```python
from build123d import *

# Parameters (mm, degrees)
SCHIZZO1_W                   = 35.5
SCHIZZO1_H                   = 64
ESTRUSIONE_ESTRUSIONE1_DEPTH = 1
SCHIZZO2_W                   = 13
SCHIZZO2_H                   = 23
ESTRUSIONE_ESTRUSIONE2_DEPTH = 2.5
SCHIZZO3_R                   = 0.51
TAGLIO_ESTRUSIONE1_DEPTH     = 2.5
ESTRUSIONE_ESTRUSIONE3_DEPTH = 7
TAGLIO_ESTRUSIONE2_DEPTH     = 6
SCHIZZO7_R                   = 1.15
TAGLIO_ESTRUSIONE3_DEPTH     = 6


with BuildPart() as part:
    # Schizzo1 → Estrusione-Estrusione1 (new body)
    with BuildSketch(Plane(origin=(0, 0, 0), x_dir=(1, 0, 0), z_dir=(0, 1, 0))):
        with Locations((-17.75, 32)):
            Rectangle(SCHIZZO1_W, SCHIZZO1_H)
    extrude(amount=ESTRUSIONE_ESTRUSIONE1_DEPTH)

    # Schizzo2 → Estrusione-Estrusione2 (add)
    with BuildSketch(Plane(origin=(0, 1, 0), x_dir=(1, 0, 0), z_dir=(0, 1, 0))):
        with Locations((-18, 60.5)):
            Rectangle(SCHIZZO2_W, SCHIZZO2_H)
    extrude(amount=ESTRUSIONE_ESTRUSIONE2_DEPTH)

    # Schizzo3 → Taglio-Estrusione1 (cut)
    with BuildSketch(Plane(origin=(0, 1, 0), x_dir=(1, 0, 0), z_dir=(0, 1, 0))):
        with Locations(Location((-1.27, 61.46, 0), (0, 0, 270))):
            Circle(SCHIZZO3_R)
        with Locations(Location((-1.27, 58.92, 0), (0, 0, 270))):
            Circle(SCHIZZO3_R)
        with Locations(Location((-1.27, 56.38, 0), (0, 0, 270))):
            Circle(SCHIZZO3_R)
        with Locations(Location((-1.27, 53.84, 0), (0, 0, 270))):
            Circle(SCHIZZO3_R)
        with Locations(Location((-1.27, 51.3, 0), (0, 0, 270))):
            Circle(SCHIZZO3_R)
        with Locations(Location((-1.27, 48.76, 0), (0, 0, 270))):
            Circle(SCHIZZO3_R)
        with Locations(Location((-1.27, 46.22, 0), (0, 0, 270))):
            Circle(SCHIZZO3_R)
        with Locations(Location((-1.27, 43.68, 0), (0, 0, 270))):
            Circle(SCHIZZO3_R)
        with Locations(Location((-1.27, 41.14, 0), (0, 0, 270))):
            Circle(SCHIZZO3_R)
        with Locations(Location((-1.27, 38.6, 0), (0, 0, 270))):
            Circle(SCHIZZO3_R)
        with Locations(Location((-1.27, 36.06, 0), (0, 0, 270))):
            Circle(SCHIZZO3_R)
        with Locations(Location((-1.27, 33.52, 0), (0, 0, 270))):
            Circle(SCHIZZO3_R)
        with Locations(Location((-1.27, 30.98, 0), (0, 0, 270))):
            Circle(SCHIZZO3_R)
        with Locations(Location((-1.27, 28.44, 0), (0, 0, 270))):
            Circle(SCHIZZO3_R)
        with Locations(Location((-1.27, 25.9, 0), (0, 0, 270))):
            Circle(SCHIZZO3_R)
        with Locations(Location((-1.27, 23.36, 0), (0, 0, 270))):
            Circle(SCHIZZO3_R)
        with Locations(Location((-1.27, 20.82, 0), (0, 0, 270))):
            Circle(SCHIZZO3_R)
        with Locations(Location((-1.27, 18.28, 0), (0, 0, 270))):
            Circle(SCHIZZO3_R)
        with Locations(Location((-1.27, 15.74, 0), (0, 0, 270))):
            Circle(SCHIZZO3_R)
        with Locations(Location((-1.27, 13.2, 0), (0, 0, 270))):
            Circle(SCHIZZO3_R)
        with Locations(Location((-34.23, 61.46, 0), (0, 0, 270))):
            Circle(SCHIZZO3_R)
        with Locations(Location((-34.23, 58.92, 0), (0, 0, 270))):
            Circle(SCHIZZO3_R)
        with Locations(Location((-34.23, 56.38, 0), (0, 0, 270))):
            Circle(SCHIZZO3_R)
        with Locations(Location((-34.23, 53.84, 0), (0, 0, 270))):
            Circle(SCHIZZO3_R)
        with Locations(Location((-34.23, 51.3, 0), (0, 0, 270))):
            Circle(SCHIZZO3_R)
        with Locations(Location((-34.23, 48.76, 0), (0, 0, 270))):
            Circle(SCHIZZO3_R)
        with Locations(Location((-34.23, 46.22, 0), (0, 0, 270))):
            Circle(SCHIZZO3_R)
        with Locations(Location((-34.23, 43.68, 0), (0, 0, 270))):
            Circle(SCHIZZO3_R)
        with Locations(Location((-34.23, 41.14, 0), (0, 0, 270))):
            Circle(SCHIZZO3_R)
        with Locations(Location((-34.23, 38.6, 0), (0, 0, 270))):
            Circle(SCHIZZO3_R)
        with Locations(Location((-34.23, 36.06, 0), (0, 0, 270))):
            Circle(SCHIZZO3_R)
        with Locations(Location((-34.23, 33.52, 0), (0, 0, 270))):
            Circle(SCHIZZO3_R)
        with Locations(Location((-34.23, 30.98, 0), (0, 0, 270))):
            Circle(SCHIZZO3_R)
        with Locations(Location((-34.23, 28.44, 0), (0, 0, 270))):
            Circle(SCHIZZO3_R)
        with Locations(Location((-34.23, 25.9, 0), (0, 0, 270))):
            Circle(SCHIZZO3_R)
        with Locations(Location((-34.23, 23.36, 0), (0, 0, 270))):
            Circle(SCHIZZO3_R)
        with Locations(Location((-34.23, 20.82, 0), (0, 0, 270))):
            Circle(SCHIZZO3_R)
        with Locations(Location((-34.23, 18.28, 0), (0, 0, 270))):
            Circle(SCHIZZO3_R)
        with Locations(Location((-34.23, 15.74, 0), (0, 0, 270))):
            Circle(SCHIZZO3_R)
        with Locations(Location((-34.23, 13.2, 0), (0, 0, 270))):
            Circle(SCHIZZO3_R)
        with Locations(Location((-21.56, 41, 0), (0, 0, 270))):
            Circle(SCHIZZO3_R)
        with Locations(Location((-19.02, 41, 0), (0, 0, 270))):
            Circle(SCHIZZO3_R)
        with Locations(Location((-16.48, 41, 0), (0, 0, 270))):
            Circle(SCHIZZO3_R)
        with Locations(Location((-13.94, 41, 0), (0, 0, 270))):
            Circle(SCHIZZO3_R)
        with Locations(Location((-28.5, 46, 0), (0, 0, 270))):
            Circle(SCHIZZO3_R)
        with Locations(Location((-25.96, 46, 0), (0, 0, 270))):
            Circle(SCHIZZO3_R)
        with Locations(Location((-23.42, 46, 0), (0, 0, 270))):
            Circle(SCHIZZO3_R)
        with Locations(Location((-28.5, 43.46, 0), (0, 0, 270))):
            Circle(SCHIZZO3_R)
        with Locations(Location((-25.96, 43.46, 0), (0, 0, 270))):
            Circle(SCHIZZO3_R)
        with Locations(Location((-23.42, 43.46, 0), (0, 0, 270))):
            Circle(SCHIZZO3_R)
    extrude(amount=-TAGLIO_ESTRUSIONE1_DEPTH, mode=Mode.SUBTRACT)

    # Schizzo6 → Estrusione-Estrusione3 (add)
    # profile 1 of 4: a face of its own
    with BuildSketch(Plane.XY):
        with BuildLine():
            Line((-26.6, 4), (-32.6, 4))
            ThreePointArc((-32.6, 4), (-34.1, 2.5), (-32.6, 1))
            Line((-32.6, 1), (-26.6, 1))
            ThreePointArc((-26.6, 1), (-25.1, 2.5), (-26.6, 4))
        make_face()
        with BuildLine():
            ThreePointArc((-32.6, 1.4), (-33.7, 2.5), (-32.6, 3.6))
            Line((-32.6, 3.6), (-26.6, 3.6))
            ThreePointArc((-26.6, 3.6), (-25.5, 2.5), (-26.6, 1.4))
            Line((-26.6, 1.4), (-32.6, 1.4))
        make_face(mode=Mode.SUBTRACT)
    # profile 2 of 4: a face of its own
    with BuildSketch(Plane.XY):
        with BuildLine():
            Line((-32.6, 1.4), (-26.6, 1.4))
            ThreePointArc((-26.6, 1.4), (-25.5, 2.5), (-26.6, 3.6))
            Line((-26.6, 3.6), (-32.6, 3.6))
            ThreePointArc((-32.6, 3.6), (-33.7, 2.5), (-32.6, 1.4))
        make_face()
    # profile 3 of 4: a face of its own
    with BuildSketch(Plane.XY):
        with BuildLine():
            ThreePointArc((-8.9, 4), (-10.4, 2.5), (-8.9, 1))
            Line((-8.9, 1), (-2.9, 1))
            ThreePointArc((-2.9, 1), (-1.4, 2.5), (-2.9, 4))
            Line((-2.9, 4), (-8.9, 4))
        make_face()
        with BuildLine():
            ThreePointArc((-8.9, 1.4), (-10, 2.5), (-8.9, 3.6))
            Line((-8.9, 3.6), (-2.9, 3.6))
            ThreePointArc((-2.9, 3.6), (-1.8, 2.5), (-2.9, 1.4))
            Line((-2.9, 1.4), (-8.9, 1.4))
        make_face(mode=Mode.SUBTRACT)
    # profile 4 of 4: a face of its own
    with BuildSketch(Plane.XY):
        with BuildLine():
            Line((-8.9, 1.4), (-2.9, 1.4))
            ThreePointArc((-2.9, 1.4), (-1.8, 2.5), (-2.9, 3.6))
            Line((-2.9, 3.6), (-8.9, 3.6))
            ThreePointArc((-8.9, 3.6), (-10, 2.5), (-8.9, 1.4))
        make_face()
    extrude(amount=-ESTRUSIONE_ESTRUSIONE3_DEPTH)

    # Schizzo6_3 → Taglio-Estrusione2 (cut)
    with BuildSketch(Plane.XY):
        with BuildLine():
            Line((-32.6, 1.4), (-26.6, 1.4))
            ThreePointArc((-26.6, 1.4), (-25.5, 2.5), (-26.6, 3.6))
            Line((-26.6, 3.6), (-32.6, 3.6))
            ThreePointArc((-32.6, 3.6), (-33.7, 2.5), (-32.6, 1.4))
        make_face()
        with BuildLine():
            Line((-8.9, 1.4), (-2.9, 1.4))
            ThreePointArc((-2.9, 1.4), (-1.8, 2.5), (-2.9, 3.6))
            Line((-2.9, 3.6), (-8.9, 3.6))
            ThreePointArc((-8.9, 3.6), (-10, 2.5), (-8.9, 1.4))
        make_face()
    extrude(amount=-TAGLIO_ESTRUSIONE2_DEPTH, mode=Mode.SUBTRACT)

    # Schizzo7 → Taglio-Estrusione3 (cut)
    with BuildSketch(Plane(origin=(0, 1, 0), x_dir=(1, 0, 0), z_dir=(0, 1, 0))):
        with Locations(Location((-29.35, 15, 0), (0, 0, 270))):
            Circle(SCHIZZO7_R)
        with Locations(Location((-6.15, 15, 0), (0, 0, 270))):
            Circle(SCHIZZO7_R)
    extrude(amount=-TAGLIO_ESTRUSIONE3_DEPTH, mode=Mode.SUBTRACT)


solid = part.part
```
Can you work these out from the model? Positions are in its coordinate system, mm. A direction names the side the tool comes from. Give positions to 0.01 mm unless a question says otherwise; leave off trailing zeros. Write each loop counter-clockwise with the first axis right and the second up, starting at its lowest first coordinate (ties: lowest second). Pieces come first, ordered by that corner, then holes. Notation, with made-up numbers: (14.5, 19.5) - (57.5, 19.5) arc R14 cw to (57.5, 40.5) - close; hole circle Ø1 at (11, -29). An arc over 180 degrees is marked (long way). Write item = value, one per line. Start each with the question number.
1. Imagine slicing it at A-A (y = 2.5). Please give me the cut outline in (x, z).
2. Thinking about a two-plate mould opening in Z: for faces 4 (the face through (-18, 0.7, 0)), 5 (the face through (-6, 3, -7)), 6 (the face through (-6.1, 0.51, -16.15)), 7 (the face through (-6, 4, -3)), which applies, released by +Z, released by -Z, zero draft, split by the parting line, or undercut?
3. For pin 1 (0.8 mm diameter, centred on x = -1.27, z = -41.14, fed in from -Y); pin 2 (1.3 mm diameter, centred on x = -1.27, z = -51.3, fed in from -Y); pin 3 (1.5 mm diameter, centred on y = 2, z = -55.5, fed in from +X); pin 4 (10 mm diameter, centred on x = -14, z = -41, fed in from +Y), each with a flat end and sliding along its axis, tell me the tip position at first contact or that it passes through.
4. On a 3-axis mill with a long thin cutter (end or side, diameter ignored), from which of +Z, -Z, +X, -X, +Y, -Y can I reach the whole of each face in a straight line? I mean faces 1 (the face through (-18, 2, -49)), 2 (the face through (-24.5, 2, -60)), 3 (the face through (-6, 3.6, -3)). Say none if no direction works.
5. Please list where these lines run through material, in increasing order: line 1 (X direction, y = 0.5, z = -25.9); line 2 (X direction, y = 0.3, z = -43.46); line 3 (X direction, y = 0.7, z = -43.68).
Worked answers:
q1.outline = (-34.1, -7) - (-25.1, -7) - (-25.1, 0) - (-25.5, 0) - (-25.5, -6) - (-33.7, -6) - (-33.7, 0) - (-34.1, 0) - close; (-24.5, -72) - (-11.5, -72) - (-11.5, -49) - (-24.5, -49) - close; (-10.4, -7) - (-1.4, -7) - (-1.4, 0) - (-1.8, 0) - (-1.8, -6) - (-10, -6) - (-10, 0) - (-10.4, 0) - close
q2.face_4 = released by +Z
q2.face_5 = released by -Z
q2.face_6 = undercut
q2.face_7 = zero draft
q3.pin_1 = through
q3.pin_2 = 0
q3.pin_3 = -11.5
q3.pin_4 = 1
q4.face_1 = +Z, +X, -X, +Y
q4.face_2 = +Z, -Z, -X, +Y
q4.face_3 = +Z
q5.line_1 = -35.5 to -34.74, -33.72 to -1.78, -0.76 to 0
q5.line_2 = -35.5 to -34.69, -33.77 to -29.01, -27.99 to -26.47, -25.45 to -23.93, -22.91 to -1.73, -0.81 to 0
q5.line_3 = -35.5 to -34.74, -33.72 to -28.96, -28.04 to -26.42, -25.5 to -23.88, -22.96 to -1.78, -0.76 to 0
